```python
from build123d import *

# Parameters (mm, degrees)
SKETCH2_W           = 2.5
SKETCH2_H           = 2.5
BOSS_EXTRUDE1_DEPTH = 7.05
PINHOLE_REACH       = 16.1
SKETCH3_W           = 0.65
SKETCH3_H           = 0.65
CUT_EXTRUDE2_DEPTH  = 0.35
SKETCH5_W           = 2.1
SKETCH5_H           = 5.3
CUT_EXTRUDE3_DEPTH  = 1.225
CUT_EXTRUDE5_DEPTH  = 0.025
SKETCH7_W           = 2.1
SKETCH7_H           = 2.1
CUT_EXTRUDE6_DEPTH  = 4
SKETCH9_W           = 0.15
SKETCH9_H           = 1
HOLDER_1_DEPTH      = 1.075
SKETCH10_W          = 1.8
SKETCH10_H          = 1
HOLDER_2_DEPTH      = 0.15


with BuildPart() as part:
    # Sketch2 → Boss-Extrude1 (new body, symmetric)
    with BuildSketch(Plane(origin=(0, 0, 0), x_dir=(1, 0, 0), z_dir=(0, 1, 0))):
        Rectangle(SKETCH2_W, SKETCH2_H)
    extrude(amount=BOSS_EXTRUDE1_DEPTH, both=True)

    # Sketch3 → Pinhole (cut, up to next)
    with BuildSketch(Plane(origin=(0, 7.05, 0), x_dir=(1, 0, 0), z_dir=(0, 1, 0)), mode=Mode.PRIVATE) as pinhole_sk1:
        Rectangle(SKETCH3_W, SKETCH3_H)
    pinhole_tool1 = extrude(pinhole_sk1.sketch, amount=-PINHOLE_REACH, mode=Mode.PRIVATE) & part.part
    add(pinhole_tool1.solids().sort_by_distance((0, 7.05, 0))[0], mode=Mode.SUBTRACT)

    # Sketch4 → Cut-Extrude2 (cut)
    with BuildSketch(Plane.XY.offset(1.25)):
        Polygon((-1.25, 3.25), (1.25, 3.25), (1.25, -2.05), (0.675, -2.05), (0.675, 1.55), (-0.675, 1.55), (-0.675, -2.05), (-1.25, -2.05), align=None)
    extrude(amount=-CUT_EXTRUDE2_DEPTH, mode=Mode.SUBTRACT)

    # Sketch5 → Cut-Extrude3 (cut)
    with BuildSketch(Plane.XY.offset(0.9)):
        with Locations((0, 0.6)):
            Rectangle(SKETCH5_W, SKETCH5_H)
    extrude(amount=-CUT_EXTRUDE3_DEPTH, mode=Mode.SUBTRACT)

    # Sketch6 → Cut-Extrude5 (cut)
    with BuildSketch(Plane.XY.offset(1.25)):
        with BuildLine():
            Line((-0.575, 0.825), (-0.575, -2.05))
            Line((-0.575, -2.05), (0.575, -2.05))
            Line((0.575, -2.05), (0.575, 0.825))
            ThreePointArc((0.575, 0.825), (0, 1.4), (-0.575, 0.825))
        make_face()
    extrude(amount=-CUT_EXTRUDE5_DEPTH, mode=Mode.SUBTRACT)

    # Sketch7 → Cut-Extrude6 (cut)
    with BuildSketch(Plane.XZ.offset(7.05)):
        Rectangle(SKETCH7_W, SKETCH7_H)
    extrude(amount=-CUT_EXTRUDE6_DEPTH, mode=Mode.SUBTRACT)

    # Sketch9 → Holder-1 (add)
    with BuildSketch(Plane.XY.offset(-0.325)):
        with Locations((-0.825, 2.4)):
            Rectangle(SKETCH9_W, SKETCH9_H)
        with Locations((0.825, 2.4)):
            Rectangle(SKETCH9_W, SKETCH9_H)
    extrude(amount=HOLDER_1_DEPTH)

    # Sketch10 → Holder-2 (add)
    with BuildSketch(Plane.XY.offset(0.75)):
        with Locations((0, 2.4)):
            Rectangle(SKETCH10_W, SKETCH10_H)
    extrude(amount=HOLDER_2_DEPTH)


solid = part.part
```
Could you check a few things on this model? Use its own coordinates, in mm. A direction names the side the tool comes from. Round coordinates to 2 decimals unless told otherwise and drop trailing zeros. Order: outer loops, then holes, each group sorted by start corner. A loop starts at its lowest first (then second) coordinate and runs counter-clockwise, first axis right, second up. Notation, with made-up numbers: (45, 49) -> (61, 49) arc R31 ccw to (61, 86) -> close; hole circle Ø4 at (84.25, 54.25). An arc over 180 degrees is marked (long way). One line per question, with ' | ' between items.
Q1. If I drill on line 1 (Y direction, x = -0.8, z = 0.2); line 2 (X direction, y = 5, z = 0.25) (3 decimals); line 3 (Y direction, x = -0.05, z = 0.7), over which ranges is the centre line in solid material (lowest first)? Write a range as from..to.
Computed values:
line 1: -3.05..-2.05, 1.9..2.9, 3.25..7.05 | line 2: -1.25..-0.325, 0.325..1.25 | line 3: -3.05..-2.05, 3.25..7.05
Q2. If we section it at B-B on x = 0: Write out the boundary of the cut face in (y, z) (3 decimals), plus the area to 3 significant figures.
Computed values:
outline: (-7.05, -1.25) -> (7.05, -1.25) -> (7.05, -0.325) -> (-3.05, -0.325) -> (-3.05, -1.05) -> (-7.05, -1.05) -> close; (-7.05, 1.05) -> (-3.05, 1.05) -> (-3.05, 0.325) -> (-2.05, 0.325) -> (-2.05, 0.9) -> (1.55, 0.9) -> (1.55, 1.25) -> (1.4, 1.25) -> (1.4, 1.225) -> (-2.05, 1.225) -> (-2.05, 1.25) -> (-7.05, 1.25) -> close; (1.9, 0.75) -> (2.9, 0.75) -> (2.9, 0.9) -> (1.9, 0.9) -> close; (3.25, 0.325) -> (7.05, 0.325) -> (7.05, 1.25) -> (3.25, 1.25) -> close | area: 16.7 mm²
Q3. If we section it at C-C on z = -0.15: Write out the boundary of the cut face in (x, y) (3 decimals), plus the area to 3 significant figures.
Computed values:
outline: (-1.25, -7.05) -> (-1.05, -7.05) -> (-1.05, -3.05) -> (-0.325, -3.05) -> (-0.325, -2.05) -> (-1.05, -2.05) -> (-1.05, 3.25) -> (-0.325, 3.25) -> (-0.325, 7.05) -> (-1.25, 7.05) -> close; (-0.9, 1.9) -> (-0.75, 1.9) -> (-0.75, 2.9) -> (-0.9, 2.9) -> close; (0.325, -3.05) -> (1.05, -3.05) -> (1.05, -7.05) -> (1.25, -7.05) -> (1.25, 7.05) -> (0.325, 7.05) -> (0.325, 3.25) -> (1.05, 3.25) -> (1.05, -2.05) -> (0.325, -2.05) -> close; (0.75, 1.9) -> (0.9, 1.9) -> (0.9, 2.9) -> (0.75, 2.9) -> close | area: 12.9 mm²
Q4. We'd pull the mould along Y, two halves only. Please class faces 1 (the face through (0, 2.4, 0.75)), 2 (the face through (1, 7.05, 0)), 3 (the face through (0.5, -3.05, 0)), 4 (the face through (1.05, -5, 0)): released by +Y, released by -Y, zero draft, split by the parting line, or undercut.
Computed values:
face 1: undercut | face 2: released by +Y | face 3: released by -Y | face 4: zero draft
Q5. If we section it at D-D on y = 5.5: Write out the boundary of the cut face in (x, z) (3 decimals).
Computed values:
outline: (-1.25, -1.25) -> (1.25, -1.25) -> (1.25, 1.25) -> (-1.25, 1.25) -> close; hole (-0.325, -0.325) -> (0.325, -0.325) -> (0.325, 0.325) -> (-0.325, 0.325) -> close
Q6. If we section it at A-A on z = 0.6: Write out the boundary of the cut face in (x, y), plus the area to 3 significant figures.
Computed values:
outline: (-1.25, -7.05) -> (-1.05, -7.05) -> (-1.05, -3.05) -> (1.05, -3.05) -> (1.05, -7.05) -> (1.25, -7.05) -> (1.25, 7.05) -> (-1.25, 7.05) -> close; (-0.9, 1.9) -> (-0.75, 1.9) -> (-0.75, 2.9) -> (-0.9, 2.9) -> close; (0.75, 1.9) -> (0.9, 1.9) -> (0.9, 2.9) -> (0.75, 2.9) -> close; hole (-1.05, -2.05) -> (1.05, -2.05) -> (1.05, 3.25) -> (-1.05, 3.25) -> close | area: 16.0 mm²
Q7. I'm going to push a flat-ended pin straight in: pin 1 (0.9 mm diameter, centred on x = 0, y = -1, fed in from +Z) (3 decimals). Where does the tip first touch, or does it pass through?
Computed values:
pin 1: z = 1.225
Q8. Which directions (+Z, -Z, +X, -X, +Y, -Y) give clear straight access to the entire face, cutting with the end or side of a thin tool? Please do faces 5 (the face through (0, 5, 1.25)), 6 (the face through (0, 0, 1.225)), 7 (the face through (-1.05, -5, 0)), 8 (the face through (0, 1, -0.325)), 9 (the face through (-1.25, 0, 0)).
Computed values:
face 5: +Z, +X, -X, +Y, -Y | face 6: +Z | face 7: -Y | face 8: none | face 9: +Z, -Z, -X, +Y, -Y
